Job drawing, mm, ordinate dimensions from the low corner. One solid piece. Round coordinates to 2 decimals unless told otherwise and drop trailing zeros. Loops run counter-clockwise (first coordinate to the right, second up) from the corner with the lowest first, then second, coordinate; pieces in that order, holes last.
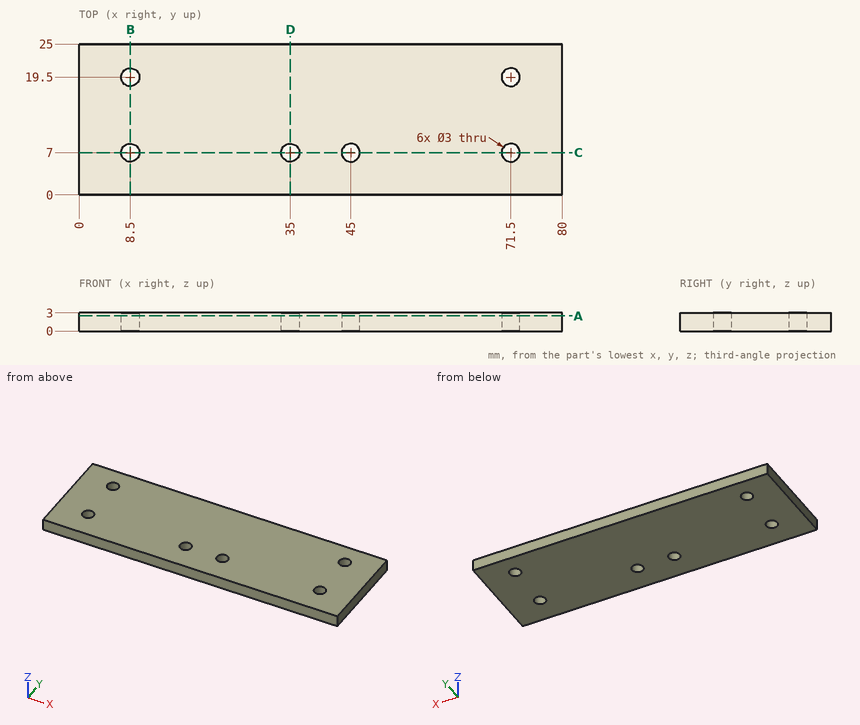
Item 1: Cut at A-A, the plane z = 2.5. Give the cut face in (x, y).
Answers follow:
outline: (0, 0) - (80, 0) - (80, 25) - (0, 25) - close; hole circle Ø3 at (8.5, 7); hole circle Ø3 at (8.5, 19.5); hole circle Ø3 at (35, 7); hole circle Ø3 at (45, 7); hole circle Ø3 at (71.5, 7); hole circle Ø3 at (71.5, 19.5)
Item 2: Cut at B-B, the plane x = 8.5. Give the cut face in (y, z), plus the area to 3 significant figures.
Answers follow:
outline: (0, 0) - (5.5, 0) - (5.5, 3) - (0, 3) - close; (8.5, 0) - (18, 0) - (18, 3) - (8.5, 3) - close; (21, 0) - (25, 0) - (25, 3) - (21, 3) - close
area: 57.0 mm2
Item 3: Cut at C-C, the plane y = 7. Give the cut face in (x, z).
Answers follow:
outline: (0, 0) - (7, 0) - (7, 3) - (0, 3) - close; (10, 0) - (33.5, 0) - (33.5, 3) - (10, 3) - close; (36.5, 0) - (43.5, 0) - (43.5, 3) - (36.5, 3) - close; (46.5, 0) - (70, 0) - (70, 3) - (46.5, 3) - close; (73, 0) - (80, 0) - (80, 3) - (73, 3) - close
Item 4: Cut at D-D, the plane x = 35. Give the cut face in (y, z).
Answers follow:
outline: (0, 0) - (5.5, 0) - (5.5, 3) - (0, 3) - close; (8.5, 0) - (25, 0) - (25, 3) - (8.5, 3) - close
Item 5: Probe line 1 (Y direction, x = 71.5, z = 0.9); line 2 (Y direction, x = 35, z = 1.2); line 3 (X direction, y = 6.25, z = 0.35). List the from-to ranges inside material, lowest first.
Answers follow:
line 1: y = 0 to 5.5, 8.5 to 18, 21 to 25
line 2: y = 0 to 5.5, 8.5 to 25
line 3: x = 0 to 7.2, 9.8 to 33.7, 36.3 to 43.7, 46.3 to 70.2, 72.8 to 80
Item 6: Flat gauge pin, fed straight in: P1, Ø1.5, axis at x = 9.5, y = 22.5, coming from the -Z side. Where does the tip first touch, or does it go through?
Answers follow:
P1: stops at z = 0
